from build123d import *

# Parameters (mm, degrees)
F0_R     = 17.125
F0_R_2   = 1.925
F1_DEPTH = 2.9
F2_R     = 3.9
F3_DEPTH = 3.75
F4_R     = 3.525
F5_DEPTH = 1.2
F4_R_2   = 3.4
F6_DEPTH = 2.6
F7_DEPTH = 25


with BuildPart() as f1:
    # F0 (on Top) → F1 (new body)
    with BuildSketch(Plane.XY):
        Circle(F0_R)
        with Locations((-7.194811, -7.194811)):
            Circle(F0_R_2, mode=Mode.SUBTRACT)
        with Locations((0, -12.975)):
            Circle(F0_R_2, mode=Mode.SUBTRACT)
        with Locations((7.194811, -7.194811)):
            Circle(F0_R_2, mode=Mode.SUBTRACT)
        with Locations((-12.975, 0)):
            Circle(F0_R_2, mode=Mode.SUBTRACT)
        with Locations((-7.194811, 7.194811)):
            Circle(F0_R_2, mode=Mode.SUBTRACT)
        with Locations((7.194811, 7.194811)):
            Circle(F0_R_2, mode=Mode.SUBTRACT)
        with Locations((12.975, 0)):
            Circle(F0_R_2, mode=Mode.SUBTRACT)
        with Locations((0, 12.975)):
            Circle(F0_R_2, mode=Mode.SUBTRACT)
    extrude(amount=F1_DEPTH)

    # F2 (on face) → F3 (join)
    with BuildSketch(Plane.XY.offset(2.9)):
        Circle(F2_R)
        Polygon((0, 2.775), (2.40322, 1.3875), (2.40322, -1.3875), (0, -2.775), (-2.40322, -1.3875), (-2.40322, 1.3875), align=None, mode=Mode.SUBTRACT)
    extrude(amount=F3_DEPTH)

    # F4 (on face) → F5 (cut)
    with BuildSketch(Plane(origin=(0, 0, 0), x_dir=(1, 0, 0), z_dir=(0, 0, -1))):
        with BuildLine():
            ThreePointArc((2.542302, -15.416787), (11.048543, -11.048543), (15.416787, -2.542302))
            ThreePointArc((15.416787, -2.542302), (12.200468, -3.438855), (9.679074, -1.25))
            Line((9.679074, -1.25), (4.841229, -1.25))
            ThreePointArc((4.841229, -1.25), (3.535534, -3.535534), (1.25, -4.841229))
            Line((1.25, -4.841229), (1.25, -9.679074))
            ThreePointArc((1.25, -9.679074), (2.901024, -10.97258), (3.525, -12.975))
            ThreePointArc((3.525, -12.975), (3.27011, -14.291057), (2.542302, -15.416787))
        make_face()
        with Locations((7.194811, -7.194811)):
            Circle(F4_R, mode=Mode.SUBTRACT)
        with BuildLine():
            ThreePointArc((9.679074, 1.25), (12.200468, 3.438855), (15.416787, 2.542302))
            ThreePointArc((15.416787, 2.542302), (11.048543, 11.048543), (2.542302, 15.416787))
            ThreePointArc((2.542302, 15.416787), (3.27011, 14.291057), (3.525, 12.975))
            ThreePointArc((3.525, 12.975), (2.901024, 10.97258), (1.25, 9.679074))
            Line((1.25, 9.679074), (1.25, 4.841229))
            ThreePointArc((1.25, 4.841229), (3.535534, 3.535534), (4.841229, 1.25))
            Line((4.841229, 1.25), (9.679074, 1.25))
        make_face()
        with Locations((7.194811, 7.194811)):
            Circle(F4_R, mode=Mode.SUBTRACT)
        with BuildLine():
            ThreePointArc((-1.25, 9.679074), (-3.438855, 12.200468), (-2.542302, 15.416787))
            ThreePointArc((-2.542302, 15.416787), (-11.048543, 11.048543), (-15.416787, 2.542302))
            ThreePointArc((-15.416787, 2.542302), (-12.200468, 3.438855), (-9.679074, 1.25))
            Line((-9.679074, 1.25), (-4.841229, 1.25))
            ThreePointArc((-4.841229, 1.25), (-3.535534, 3.535534), (-1.25, 4.841229))
            Line((-1.25, 4.841229), (-1.25, 9.679074))
        make_face()
        with Locations((-7.194811, 7.194811)):
            Circle(F4_R, mode=Mode.SUBTRACT)
        with BuildLine():
            ThreePointArc((-15.416787, -2.542302), (-11.048543, -11.048543), (-2.542302, -15.416787))
            ThreePointArc((-2.542302, -15.416787), (-3.438855, -12.200468), (-1.25, -9.679074))
            Line((-1.25, -9.679074), (-1.25, -4.841229))
            ThreePointArc((-1.25, -4.841229), (-3.535534, -3.535534), (-4.841229, -1.25))
            Line((-4.841229, -1.25), (-9.679074, -1.25))
            ThreePointArc((-9.679074, -1.25), (-12.200468, -3.438855), (-15.416787, -2.542302))
        make_face()
        with Locations((-7.194811, -7.194811)):
            Circle(F4_R, mode=Mode.SUBTRACT)
    extrude(amount=-F5_DEPTH, mode=Mode.SUBTRACT)

    # F4 (on face) → F6 (cut)
    with BuildSketch(Plane(origin=(0, 0, 0), x_dir=(1, 0, 0), z_dir=(0, 0, -1))):
        Circle(F4_R_2)
        Polygon((0, 1.9), (1.645448, 0.95), (1.645448, -0.95), (0, -1.9), (-1.645448, -0.95), (-1.645448, 0.95), align=None, mode=Mode.SUBTRACT)
    extrude(amount=-F6_DEPTH, mode=Mode.SUBTRACT)

    # F4 (on face) → F7 (cut)
    with BuildSketch(Plane(origin=(0, 0, 0), x_dir=(1, 0, 0), z_dir=(0, 0, -1))):
        Polygon((1.645448, -0.95), (1.645448, 0.95), (0, 1.9), (-1.645448, 0.95), (-1.645448, -0.95), (0, -1.9), align=None)
    extrude(amount=-F7_DEPTH, mode=Mode.SUBTRACT)


solid = f1.part
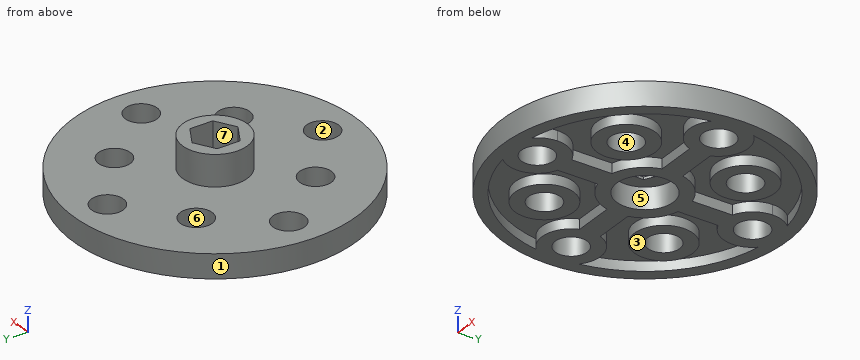
Geometry: final body of the model. Coordinates: model frame, mm. Face numbers are marked on the shaded views. A direction names the side the tool comes from. Round coordinates to 2 decimals unless told otherwise and drop trailing zeros. Order: outer loops, then holes, each group sorted by start corner. A loop starts at its lowest first (then second) coordinate and runs counter-clockwise, first axis right, second up.
Q1. Pin query (flat end, axial travel): pin 1 (0.8 mm diameter, centred on y = -0.5, z = 4.5, fed in from +X); pin 2 (0.8 mm diameter, centred on y = -0.5, z = 4.5, fed in from -X); pin 3 (2 mm diameter, centred on y = 4, z = 4, fed in from -X). Return the tip coordinate at first contact, or that it passes through.
Result sheet:
pin 1: stops at x = 3.9
pin 2: stops at x = -3.9
pin 3: stops at x = -2.49
Q2. Section B-B, the plane x = -13.5. Output: boundary loops of the cut face in (y, z), and give its area (3 significant figures).
Result sheet:
outline: (-10.54, 0) - (-7.87, 0) - (-7.87, 1.2) - (-3.49, 1.2) - (-3.49, 0) - (-1.85, 0) - (-1.85, 2.9) - (-10.54, 2.9) - close; (1.85, 0) - (3.49, 0) - (3.49, 1.2) - (7.87, 1.2) - (7.87, 0) - (10.54, 0) - (10.54, 2.9) - (1.85, 2.9) - close
area: 39.9 mm2
Q3. Section D-D, the plane x = 14.5. Output: boundary loops of the cut face in (y, z), and give its area (3 significant figures).
Result sheet:
outline: (-9.11, 0) - (-5.82, 0) - (-5.82, 1.2) - (-3.18, 1.2) - (-3.18, 0) - (-1.17, 0) - (-1.17, 2.9) - (-9.11, 2.9) - close; (1.17, 0) - (3.18, 0) - (3.18, 1.2) - (5.82, 1.2) - (5.82, 0) - (9.11, 0) - (9.11, 2.9) - (1.17, 2.9) - close
area: 39.7 mm2
Q4. Access query for the marked faces 5, 6 and 7. Directions: +Z, -Z, +X, -X, +Y, -Y. A direction counts if a zero-diameter tool reaches every point of the face in a straight line with its end or side. Return the directions, or none.
Result sheet:
face 5: -Z
face 6: +Z, -Z
face 7: +Z
Q5. Section A-A, the plane y = 0. Output: boundary loops of the cut face in (x, z) (3 decimals), and give its area (3 significant figures).
Result sheet:
outline: (-17.125, 0) - (-14.9, 0) - (-14.9, 2.9) - (-17.125, 2.9) - close; (-11.05, 0) - (-3.4, 0) - (-3.4, 2.6) - (-1.645, 2.6) - (-1.645, 2.9) - (-2.403, 2.9) - (-2.403, 6.65) - (-3.9, 6.65) - (-3.9, 2.9) - (-11.05, 2.9) - close; (1.645, 2.6) - (3.4, 2.6) - (3.4, 0) - (11.05, 0) - (11.05, 2.9) - (3.9, 2.9) - (3.9, 6.65) - (2.403, 6.65) - (2.403, 2.9) - (1.645, 2.9) - close; (14.9, 0) - (17.125, 0) - (17.125, 2.9) - (14.9, 2.9) - close
area: 69.6 mm2
Q6. Material intervals for probe 1 along Y at (x, z) = (0, 0.75) (3 decimals); probe 2 along X at (y, z) = (-8.5, 1.75); probe 3 along Y at (x, z) = (-4, 0.75), sorted ascending.
Result sheet:
probe 1: y = -17.125 to -14.9, -11.05 to -3.4, 3.4 to 11.05, 14.9 to 17.125
probe 2: x = -14.87 to -8.61, -5.78 to 5.78, 8.61 to 14.87
probe 3: y = -16.65 to -15.1, -8.68 to -5.71, -3 to 3, 5.71 to 8.68, 15.1 to 16.65
Q7. Mould query, pull axis Y, two halves, no side actions, for the marked faces 1, 2, 3 and 4. Classes: released by +Y, released by -Y, zero draft, split by the parting line, or undercut.
Result sheet:
face 1: split by the parting line
face 2: undercut
face 3: zero draft
face 4: undercut
Q8. Section C-C, the plane y = 8.5. Output: boundary loops of the cut face in (x, z).
Result sheet:
outline: (-14.87, 0) - (-13.11, 0) - (-13.11, 1.2) - (-10.47, 1.2) - (-10.47, 0) - (-8.61, 0) - (-8.61, 2.9) - (-14.87, 2.9) - close; (-5.78, 0) - (-3.92, 0) - (-3.92, 1.2) - (-1.25, 1.2) - (-1.25, 0) - (1.25, 0) - (1.25, 1.2) - (3.92, 1.2) - (3.92, 0) - (5.78, 0) - (5.78, 2.9) - (-5.78, 2.9) - close; (8.61, 0) - (10.47, 0) - (10.47, 1.2) - (13.11, 1.2) - (13.11, 0) - (14.87, 0) - (14.87, 2.9) - (8.61, 2.9) - close
